Part print with two shaded views. Sizes in mm from the minimum x, y, z corner. Give positions to 0.01 mm unless a question says otherwise; leave off trailing zeros. Write each loop counter-clockwise with the first axis right and the second up, starting at its lowest first coordinate (ties: lowest second). Pieces come first, ordered by that corner, then holes. Notation, with made-up numbers: M -0.5,47.25 L 39.5,47.25 A19 ccw 39.5,72.25 Z; hole C -5.5,61 d11. An arc over 180 degrees is marked long. Return JSON: item names as keys, results as strings. Group by question number.
Q1. Wall check: probe 1 along X at (y, z) = (7.75, 80); probe 2 along Z at (x, y) = (39, 1); probe 3 along Z at (x, y) = (32, 4.5). Give the ranges that are in metal, low to high.
Q2. Band-saw the part on C-C, the plane y = 6.75. Give the cut face in (x, z) (1 decimal).
Q3. Flat gauge pin, fed straight in: pin 1 Ø5 at (x, y) = (36, 8) entering from +Z. Where does the tip first touch, or does it go through?
Q4. Band-saw the part on B-B, the plane x = 25. Give the cut face in (y, z) (1 decimal), then the cut area to 3 significant figures.
Q5. Band-saw the part on D-D, the plane x = 5. Give the cut face in (y, z), then the cut area to 3 significant figures.
Q6. Band-saw the part on A-A, the plane z = 80. Give the cut face in (x, y), then the cut area to 3 significant figures.
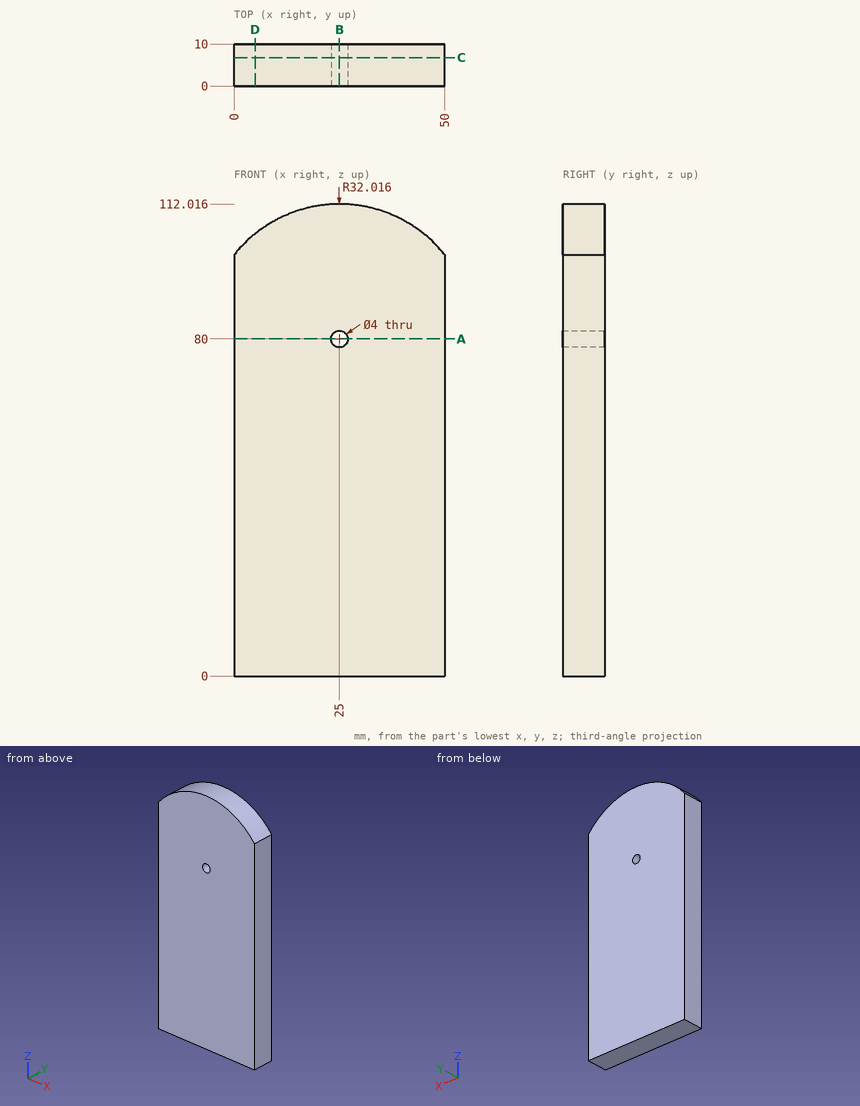
From the geometry:
{
 "1": {"probe 1": "x = 0 to 23, 27 to 50", "probe 2": "z = 0 to 108.79", "probe 3": "z = 0 to 111.24"},
 "2": {"outline": "M 0,0 L 50,0 L 50,100 A32 ccw 0,100 Z; hole C 25,80 d4"},
 "3": {"pin 1": "stops at z = 110.87"},
 "4": {"outline": "M 0,0 L 10,0 L 10,78 L 0,78 Z; M 0,82 L 10,82 L 10,112 L 0,112 Z", "area": "1,080 mm^2"},
 "5": {"outline": "M 0,0 L 10,0 L 10,105 L 0,105 Z", "area": "1,050 mm^2"},
 "6": {"outline": "M 0,0 L 23,0 L 23,10 L 0,10 Z; M 27,0 L 50,0 L 50,10 L 27,10 Z", "area": "460 mm^2"}
}
